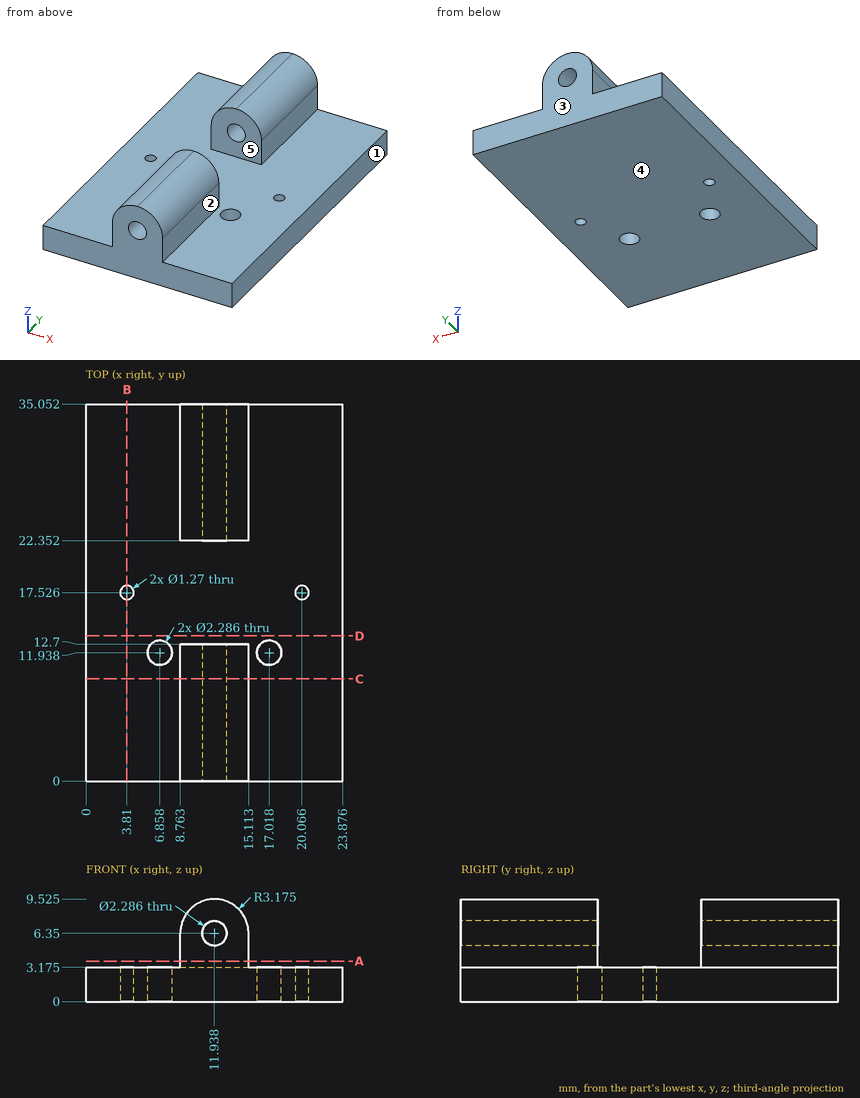
Source: three-view drawing plus pictorial views. Frame: mm from the lowest corner of the part. A direction names the side the tool comes from. Round coordinates to 2 decimals unless told otherwise and drop trailing zeros. Loops run counter-clockwise (first coordinate to the right, second up) from the corner with the lowest first, then second, coordinate; pieces in that order, holes last.
Q1. Material intervals for L1, parallel to Y at x = 7, z = 2.75; L2, parallel to Y at x = 12.75, z = 5.5; L3, parallel to Z at x = 20.5, y = 31 (3 decimals), sorted ascending.
Q2. Pin query (flat end, axial travel): P1, Ø1.7, axis at x = 3.81, y = 17.526, coming from the +Z side (3 decimals); P2, Ø1, axis at y = 32, z = 5, coming from the -X side; P3, Ø2.5, axis at y = 30.5, z = 5, coming from the +X side. Return the tip coordinate at first contact, or that it passes through.
Q3. Section D-D on y = 13.5. Return loops of the section in (x, z) (3 decimals).
Q4. Section B-B on x = 3.81. Return loops of the section in (y, z) (3 decimals), plus the area to 3 significant figures.
Q5. Pull-direction query (Y, two-part tool) for the marked faces 3, 4 and 5; classes: released by +Y, released by -Y, zero draft, split by the parting line, or undercut.
Q6. Section A-A on z = 3.75. Return loops of the section in (x, y), plus the area to 3 significant figures.
Q7. Access query for the marked faces 1 and 2. Directions: +Z, -Z, +X, -X, +Y, -Y. A direction counts if a zero-diameter tool reaches every point of the face in a straight line with its end or side. Return the directions, or none.
Q8. Section C-C on y = 9.5. Return loops of the section in (x, z) (3 decimals).
Evaluation:
1. L1: y = 0 to 10.8, 13.07 to 35.05
1. L2: y = 0 to 12.7, 22.35 to 35.05
1. L3: z = 0 to 3.175
2. P1: stops at z = 3.175
2. P2: stops at x = 8.76
2. P3: stops at x = 15.11
3. outline: (0, 0) - (23.876, 0) - (23.876, 3.175) - (0, 3.175) - close
4. outline: (0, 0) - (16.891, 0) - (16.891, 3.175) - (0, 3.175) - close; (18.161, 0) - (35.052, 0) - (35.052, 3.175) - (18.161, 3.175) - close
4. area: 107 mm2
5. face 3: released by +Y
5. face 4: zero draft
5. face 5: undercut
6. outline: (8.76, 0) - (15.11, 0) - (15.11, 12.7) - (8.76, 12.7) - close; (8.76, 22.35) - (15.11, 22.35) - (15.11, 35.05) - (8.76, 35.05) - close
6. area: 161 mm2
7. face 1: +Z, -Z, +X, +Y, -Y
7. face 2: +Z, +X, +Y, -Y
8. outline: (0, 0) - (23.876, 0) - (23.876, 3.175) - (15.113, 3.175) - (15.113, 6.35) arc R3.175 ccw to (8.763, 6.35) - (8.763, 3.175) - (0, 3.175) - close; hole circle Ø2.286 at (11.938, 6.35)
